The model under review builds one solid part; all positions refer to its coordinate system, in mm. Round coordinates to 2 decimals unless told otherwise and drop trailing zeros. Order: outer loops, then holes, each group sorted by start corner. A loop starts at its lowest first (then second) coordinate and runs counter-clockwise, first axis right, second up. Notation, with made-up numbers: (-0.5, -28) -> (53.5, -28) arc R32 cw to (53.5, 7) -> close; hole circle Ø11 at (17.5, -5). An arc over 180 degrees is marked (long way). Put each result on its own line as item: value. Start each with the question number.
Autodesk Inventor part; units mm, degrees
ref_plane "YZ Plane" through (0, 0, 0) normal (1, 0, 0) x (0, 1, 0)
ref_plane "XZ Plane" through (0, 0, 0) normal (0, 1, 0) x (-1, 0, 0)
ref_plane "XY Plane" through (0, 0, 0) normal (0, 0, 1) x (1, 0, 0)
sketch "Sketch1" plane through (0, 0, 0) normal (1, 0, 0) x (0, 1, 0)
  line L0 (20, 10) -> (-30, 10)
  line L1 (-30, 10) -> (-30, -10)
  line L2 (-30, -10) -> (20, -10)
  arc A0 (20, -10) -> (20, 10) centre (20, 0) ccw
  circle A1 centre (20, 0) radius 2.5
  point P0 (0, 0)
extrude "Extrusion1" add sketch "Sketch1" along normal blind 3
properties part number "Conveyor Stand" material "Pine, Southern"
Q1. Wall thickness on probe 1 along Z at (x, y) = (1.45, 20); probe 2 along Y at (x, z) = (2.25, -1.25); probe 3 along Y at (x, z) = (2.1, 1.75): over which ranges is each line inside the solid? List them lowest first. Write a range as [from, to].
Q2. Take a section at D-D on z = -7. Give the boundary of the cut face in (x, y), and give its area (3 significant figures).
Q3. Take a section at B-B on x = 2.5. Give the boundary of the cut face in (y, z), and give its area (3 significant figures).
Q4. Take a section at C-C on z = 8.75. Give the boundary of the cut face in (x, y), and give its area (3 significant figures).
Q5. Draft analysis for pull direction Y (two halves, no side actions). For faces 1 (the face through (1, 30, 0)), 2 (the face through (1, -5, -10)), 3 (the face through (1.5, 17.5, -0.1)), 4 (the face through (1, -30, 0)), state which applies: +Y half, -Y half, draft (parallel to the pull), parting line (faces both ways), or undercut.
Q6. Take a section at A-A on z = 0. Give the boundary of the cut face in (x, y).
Calculated:
1. probe 1: z = [-10, -2.5], [2.5, 10]
1. probe 2: y = [-30, 17.83], [22.17, 29.92]
1. probe 3: y = [-30, 18.21], [21.79, 29.85]
2. outline: (0, -30) -> (3, -30) -> (3, 27.14) -> (0, 27.14) -> close
2. area: 171 mm²
3. outline: (-30, -10) -> (20, -10) arc R10 ccw to (20, 10) -> (-30, 10) -> close; hole circle Ø5 at (20, 0)
3. area: 1,140 mm²
4. outline: (0, -30) -> (3, -30) -> (3, 24.84) -> (0, 24.84) -> close
4. area: 165 mm²
5. face 1: +Y half
5. face 2: draft
5. face 3: undercut
5. face 4: -Y half
6. outline: (0, -30) -> (3, -30) -> (3, 17.5) -> (0, 17.5) -> close; (0, 22.5) -> (3, 22.5) -> (3, 30) -> (0, 30) -> close
